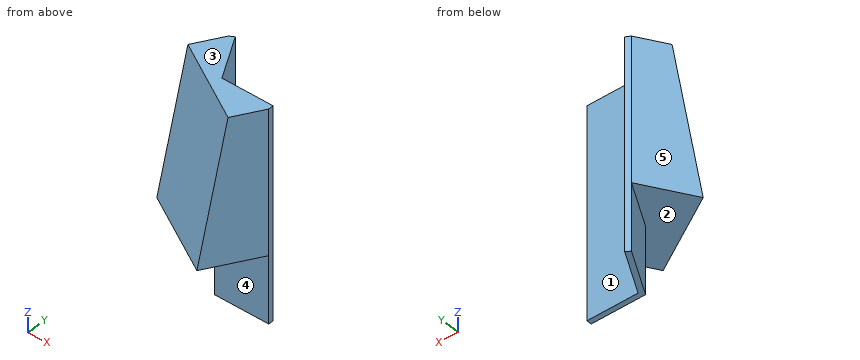
```python
from build123d import *

# Parameters (mm, degrees)
BOSS_EXTRUDE2_DEPTH      = 80
BOSS_EXTRUDE3_DEPTH      = 18.320508
BOSS_EXTRUDE3_DEPTH_BACK = 18.320508
BOSS_EXTRUDE4_REACH      = 87.413
SKETCH6_W                = 54.567226391
SKETCH6_H                = 16.588457268
BOSS_EXTRUDE5_REACH      = 87.413
SKETCH8_W                = 16.588457268
SKETCH8_H                = 54.567226391


with BuildPart() as part:
    # Sketch3 → Boss-Extrude2 (new body)
    with BuildSketch(Plane.XY):
        Polygon((0, 0), (-10.577350269, 18.320508076), (-8.845299462, 19.320508076), (1.154700538, 2), (21.154700538, 2), (21.154700538, 0), align=None)
    extrude(amount=BOSS_EXTRUDE2_DEPTH)

    # Sketch5 → Boss-Extrude3 (add, two sides: drawn at the far end of the back side and taken through both)
    with BuildSketch(Plane(origin=(0, 0, 0), x_dir=(0, 0, -1), z_dir=(0.86602540378444, -0.4999999999999977, 0)).offset(-BOSS_EXTRUDE3_DEPTH_BACK)):
        Polygon((-25.432773609, -9.621674275), (-25.432773609, -11.621674275), (-80, -2), (-80, 0), (-80, 1), (-25.432773609, 1), (-25.432773609, 0), align=None)
    extrude(amount=BOSS_EXTRUDE3_DEPTH + BOSS_EXTRUDE3_DEPTH_BACK)

    # Sketch6 → Boss-Extrude4 (add, up to next)
    with BuildSketch(Plane(origin=(0.4999999999999976, 0.8660254037844397, 0), x_dir=(0, 0, -1), z_dir=(0.49999999999999784, 0.8660254037844398, 0)), mode=Mode.PRIVATE) as boss_extrude4_sk1:
        with Locations((-52.716386805, 10.026279442)):
            Rectangle(SKETCH6_W, SKETCH6_H)
    boss_extrude4_tool1 = extrude(boss_extrude4_sk1.sketch, amount=BOSS_EXTRUDE4_REACH, mode=Mode.PRIVATE) - part.part
    add(boss_extrude4_tool1.solids().sort_by_distance((-8.183013, 5.879165, 52.716387))[0])

    # Sketch8 → Boss-Extrude5 (add, up to next)
    with BuildSketch(Plane(origin=(0.4999999999999976, 0.8660254037844397, 0), x_dir=(0.8660254037844399, -0.4999999999999979, 0), z_dir=(0.49999999999999784, 0.8660254037844398, 0)), mode=Mode.PRIVATE) as boss_extrude5_sk1:
        with Locations((10.026279442, -52.716386805)):
            Rectangle(SKETCH8_W, SKETCH8_H)
    boss_extrude5_tool1 = extrude(boss_extrude5_sk1.sketch, amount=BOSS_EXTRUDE5_REACH, mode=Mode.PRIVATE) - part.part
    add(boss_extrude5_tool1.solids().sort_by_distance((9.183013, -4.147114, 52.716387))[0])


solid = part.part
```
For this review, take the finished solid that the model builds, in its own axes (mm). Face numbers are marked on the shaded views. A direction names the side the tool comes from. Round coordinates to 2 decimals unless told otherwise and drop trailing zeros. Loops run counter-clockwise (first coordinate to the right, second up) from the corner with the lowest first, then second, coordinate; pieces in that order, holes last.
Q1. Add section B-B on z = 22.5. Write out the cut boundary in (x, y).
Result sheet:
outline: (-10.58, 18.32) - (0, 0) - (21.15, 0) - (21.15, 2) - (1.15, 2) - (-8.85, 19.32) - close
Q2. Add section C-C on y = 4.5. Write out the cut boundary in (x, z), plus the area to 3 significant figures.
Result sheet:
outline: (-18.56, 25.43) - (-2.6, 25.43) - (-2.6, 0) - (-0.29, 0) - (-0.29, 80) - (-11.79, 80) - (-18.56, 60.82) - close
area: 991 mm2
Q3. Insertion check: pin 1 Ø2 at (x, z) = (1.5, 13.5) entering from +Y; pin 2 Ø4 at (x, z) = (3.5, 48.5) entering from -Y; pin 3 Ø5 at (y, z) = (7, 58) entering from -X. Each pin has a flat end and moves straight along its axis. Give the tip position at first contact, or say it passes through.
Result sheet:
pin 1: stops at y = 3.13
pin 2: stops at y = -11.97
pin 3: stops at x = -18.56
Q4. To check wall thickness, follow line 1 along Z through (x, y) = (12.5, -5); line 2 along Y through (x, z) = (8, 20.5); line 3 along Y through (x, z) = (17.5, 28.5). State the ranges of each line that lie inside material, in increasing order.
Result sheet:
line 1: z = 25.43 to 80
line 2: y = 0 to 2
line 3: y = -6.33 to 2
Q5. Add section D-D on y = 13. Write out the cut boundary in (x, z).
Result sheet:
outline: (-13.65, 25.43) - (-7.51, 25.43) - (-7.51, 0) - (-5.2, 0) - (-5.2, 80) - (-13.65, 80) - close
Q6. Machinability: for the marked faces 1, 2, 3, 4 and 5, which of the approach directions +Z, -Z, +X, -X, +Y, -Y give a long, thin tool a straight path to every point of the face, cutting with its end or side? Answer none if there is none.
Result sheet:
face 1: +Z, -Z, +X, +Y
face 2: -Z, -X, -Y
face 3: +Z, +X, -X, +Y, -Y
face 4: -Z, +X, -X, -Y
face 5: +Z, -Z, -X, +Y
Q7. Add section A-A on x = 14. Write out the cut boundary in (y, z), plus the area to 3 significant figures.
Result sheet:
outline: (-12.39, 25.43) - (0, 25.43) - (0, 0) - (2, 0) - (2, 80) - (-10.39, 80) - (-12.39, 70.18) - close
area: 826 mm2
